Here's how the part is built. I have some questions about the finished solid (model axes, mm). A direction names the side the tool comes from. Give positions to 0.01 mm unless a question says otherwise; leave off trailing zeros. Order: outer loops, then holes, each group sorted by start corner. A loop starts at its lowest first (then second) coordinate and runs counter-clockwise, first axis right, second up. Notation, with made-up numbers: M 18,76.25 L 41,76.25 A13 cw 41,87.25 Z; hole C -8,15.25 d4. An arc over 180 degrees is marked long. Use one line per item in the form item = value.
from build123d import *

# Parameters (mm, degrees)
PAD_DEPTH    = 20
FILLET_R     = 4.5
SKETCH001_R  = 2.5
PAD001_DEPTH = 5
PAD002_DEPTH = 3


with BuildPart() as part:
    # Sketch → Pad (new body)
    with BuildSketch(Plane.XY):
        Polygon((0, -2.5), (0, -6), (10, -6), (10, 6), (0, 6), (0, 2.5), align=None)
    extrude(amount=PAD_DEPTH)

    # Fillet
    fillet_edges = [part.edges().sort_by_distance(p)[0] for p in [
        (10, -6, 10),
        (10, 6, 10),
    ]]
    fillet(fillet_edges, radius=FILLET_R)

    # Sketch001 → Pad001 (join)
    with BuildSketch(Plane.YZ):
        with Locations((0, 6.466317)):
            Circle(SKETCH001_R)
    extrude(amount=-PAD001_DEPTH)

    # Sketch002 → Pad002 (join)
    with BuildSketch(Plane(origin=(-4, 0, 0), x_dir=(0, 0.838671, 0.544639), z_dir=(1, 0, 0))):
        with BuildLine():
            ThreePointArc((6.72858, 2.526992), (9.504552, 4.716507), (7.315037, 7.49248))
            Line((7.315037, 7.49248), (0.315037, 8.319227))
            ThreePointArc((0.315037, 8.319227), (-2.460935, 6.129712), (-0.27142, 3.353739))
            Line((6.72858, 2.526992), (-0.27142, 3.353739))
        make_face()
    extrude(amount=-PAD002_DEPTH)


solid = part.part
Q1. Thinking about a two-plate mould opening in X: for faces 4 (the face through (8.717, 4.647, 10.14)), 5 (the face through (-1.909, -0.325, 8.945)), 6 (the face through (-5.48, -1.06, 8.73)), which applies, +X half, -X half, draft (parallel to the pull), parting line (faces both ways), or undercut?
Found:
face_4 = +X half
face_5 = undercut
face_6 = draft
Q2. I want a section at D-D on y = 0. Write out the boundary of the cut face in (x, z).
Found:
outline = M -7,3.68 L -4,3.68 L -4,3.97 L 0,3.97 L 0,0 L 10,0 L 10,20 L 0,20 L 0,8.97 L -4,8.97 L -4,9.25 L -7,9.25 Z
Q3. I'm going to push flat-ended pins straight in: pin 1 Ø1.5 at (y, z) = (4, 17.5) entering from -X; pin 2 Ø1.5 at (x, y) = (-3.5, -2) entering from +Z. Where does each tip first touch, or does it pass through?
Found:
pin_1 = 0
pin_2 = 8.63
Q4. On a 3-axis mill with a long thin cutter (end or side, diameter ignored), from which of +Z, -Z, +X, -X, +Y, -Y can I reach the whole of each face in a straight line? I mean faces 1 (the face through (-5.479, 1.151, 4.246)), 2 (the face through (-4, 1.8, 8.5)), 3 (the face through (10, 0, 10)). Say none if no direction works.
Found:
face_1 = -Z, -X, +Y
face_2 = none
face_3 = +Z, -Z, +X, +Y, -Y
Q5. I want a section at C-C on x = -5.5. Write out the boundary of the cut face in (y, z), then the cut area to 3 significant figures.
Found:
outline = M -4.27,7.15 A2.5 ccw -2.05,2.66 L 4.27,5.78 A2.5 ccw 2.05,10.27 Z
area = 54.9 mm²
Q6. I want a section at A-A on y = -3. Write out the boundary of the cut face in (x, z).
Found:
outline = M -7,2.41 L -4,2.41 L -4,7.77 L -7,7.77 Z; M 0,0 L 9.74,0 L 9.74,20 L 0,20 Z
Q7. I need wall thicknesses on L1, parallel to X at y = 3.25, z = 8.5; L2, parallel to X at y = -1, z = 13.5; L3, parallel to Y at x = -2, z = 4.5. Which ranges of each line are inside material? Lowest first, please.
Found:
L1 = -7 to -4, 0 to 9.65
L2 = 0 to 10
L3 = -1.54 to 1.54
Q8. I want a section at B-B on z = 11.25. Write out the boundary of the cut face in (x, y), then the cut area to 3 significant figures.
Found:
outline = M 0,-6 L 5.5,-6 A4.5 ccw 10,-1.5 L 10,1.5 A4.5 ccw 5.5,6 L 0,6 Z
area = 111 mm²
